The listing builds one solid part. Answer for the finished solid, in the listing's coordinates (mm). Face numbers are marked on the shaded views. A direction names the side the tool comes from. Give positions to 0.01 mm unless a question says otherwise; leave off trailing zeros. Write each loop counter-clockwise with the first axis right and the second up, starting at its lowest first coordinate (ties: lowest second). Pieces come first, ordered by that corner, then holes. Notation, with made-up numbers: (-1, -26) - (55, -26) arc R27 cw to (55, 3) - close; hole circle Ø1 at (-25.5, 80.25). An arc over 180 degrees is marked (long way). Answer as CSV lines item,"result". Start each with the question number.
(1) Find section B-B (z = 0). Write down the section's boundary in (x, y) (3 decimals), then the cut area to 3 significant figures.
(2) Straight lines are drawn through the part: probe 1 along Z at (x, y) = (-0.5, -4); probe 2 along X at (y, z) = (-6.5, 0); probe 3 along X at (y, z) = (108.73, 17.25). For each, find the intervals that lie inside material, in ascending order.
(3) Each of these flat-tipped pins is pushed along its axis until it touches: pin 1 Ø2.5 at (x, z) = (-20, -28) entering from -Y; pin 2 Ø1 at (x, z) = (14, -2.5) entering from +Y; pin 3 Ø17 at (y, z) = (89.5, 13.5) entering from +X. Where does it stop, or does it pass through?
(4) For a pull along Y with two mould halves and no side action, classify the marked faces 6, 7 and 8 as pulls with the +Y half, pulls with the -Y half, needs draft (parallel to the pull), parting line crosses it, or undercut.
(5) For the marked faces 1, 2, 3, 4 and 5, determine the directions among +Z, -Z, +X, -X, +Y, -Y from which every point of the face is accessible in a straight line to the end or side of a thin tool.
(6) Find section D-D (y = 3). Write down the section's boundary in (x, z).
(7) Find section C-C (y = 28.5). Write down the section's boundary in (x, z).
(8) Find section A-A (z = -30.68). Write down the section's boundary in (x, y).
from build123d import *

# Parameters (mm, degrees)
SKETCH_1_R           = 20.68
SKETCH_1_R_2         = 9.68
EXTRUDE_1_DEPTH      = 116.68
SKETCH_11_W          = 27
SKETCH_11_H          = 150
CUT_EXTRUDE_3_DEPTH  = 40
SKETCH_13_W          = 10
SKETCH_13_H          = 128.345013401
CUT_EXTRUDE_7_DEPTH  = 126.614916312
SKETCH_15_W          = 8
SKETCH_15_H          = 68.68
CUT_EXTRUDE_9_DEPTH  = 48
SKETCH_16_W          = 15.549431524
SKETCH_16_H          = 20
SKETCH_16_W_2        = 15.459431524
EXTRUDE_4_DEPTH      = 19.2
SKETCH_17_W          = 19.20851187
SKETCH_17_H          = 14.03
CUT_EXTRUDE_10_DEPTH = 20.2
SKETCH_18_R          = 9.59
CUT_EXTRUDE_11_DEPTH = 121.289430957
SKETCH_21_R          = 2.985
CUT_EXTRUDE_12_DEPTH = 55.2
EXTRUDE_START        = 55.2
SKETCH_24_R          = 20.59
SKETCH_24_R_2        = 9.59
EXTRUDE_2_DEPTH      = 55.2
CUT_EXTRUDE_13_DEPTH = 55.2
SKETCH_26_W          = 10.00851187
SKETCH_26_H          = 41.68
CUT_EXTRUDE_15_DEPTH = 55.2
SKETCH_27_W          = 10
SKETCH_27_H          = 40
CUT_EXTRUDE_16_DEPTH = 55.2
SKETCH_28_W          = 44.880694938
SKETCH_28_H          = 9.608044066
CUT_EXTRUDE_17_DEPTH = 12.2
SKETCH_35_W          = 13.53
SKETCH_35_H          = 20
EXTRUDE_10_DEPTH     = 15
EXTRUDE_11_DEPTH     = 15
SKETCH_37_W          = 9
SKETCH_37_H          = 20
EXTRUDE_12_DEPTH     = 20
SKETCH_38_W          = 9
SKETCH_38_H          = 20
EXTRUDE_13_DEPTH     = 20
SKETCH_42_R          = 2.985
CUT_EXTRUDE_21_DEPTH = 20


with BuildPart() as part:
    # 草圖1 → 伸長-薄件1 (new body)
    with BuildSketch(Plane(origin=(0, 0, 0), x_dir=(1, 0, 0), z_dir=(0, 1, 0))):
        Circle(SKETCH_1_R)
        Circle(SKETCH_1_R_2, mode=Mode.SUBTRACT)
    extrude(amount=EXTRUDE_1_DEPTH)

    # 草圖11 → 除料-伸長3 (cut)
    with BuildSketch(Plane(origin=(0, 116.68, 0), x_dir=(1, 0, 0), z_dir=(0, 1, 0))):
        with Locations((21.70851187, -44.235815192)):
            Rectangle(SKETCH_11_W, SKETCH_11_H)
    extrude(amount=-CUT_EXTRUDE_3_DEPTH, mode=Mode.SUBTRACT)

    # 草圖13 → 除料-伸長7 (cut, through all)
    with BuildSketch(Plane.XY.offset(21)):
        with Locations((-16, 58.612182466)):
            Rectangle(SKETCH_13_W, SKETCH_13_H)
    extrude(amount=-CUT_EXTRUDE_7_DEPTH, mode=Mode.SUBTRACT)

    # 草圖15 → 除料-伸長9 (cut)
    with BuildSketch(Plane.XY.offset(21)):
        with Locations((-1.395744065, 52.34)):
            Rectangle(SKETCH_15_W, SKETCH_15_H)
    extrude(amount=-CUT_EXTRUDE_9_DEPTH, mode=Mode.SUBTRACT)

    # 草圖16 → 填料-伸長4 (add)
    with BuildSketch(Plane(origin=(8.20851187, 0, 0), x_dir=(0, 0, -1), z_dir=(1, 0, 0))):
        with Locations((12.905284238, 106.68)):
            Rectangle(SKETCH_16_W, SKETCH_16_H)
        with Locations((-12.860284238, 106.68)):
            Rectangle(SKETCH_16_W_2, SKETCH_16_H)
    extrude(amount=-EXTRUDE_4_DEPTH)

    # 草圖17 → 除料-伸長10 (cut)
    with BuildSketch(Plane(origin=(0, 116.68, 0), x_dir=(1, 0, 0), z_dir=(0, 1, 0))):
        with Locations((-1.395744065, -0.045)):
            Rectangle(SKETCH_17_W, SKETCH_17_H)
    extrude(amount=-CUT_EXTRUDE_10_DEPTH, mode=Mode.SUBTRACT)

    # 草圖18 → 除料-伸長11 (cut, through all)
    with BuildSketch(Plane.XZ):
        with Locations(Location((0, 0, 0), (0, 0, 90))):
            Circle(SKETCH_18_R)
    extrude(amount=-CUT_EXTRUDE_11_DEPTH, mode=Mode.SUBTRACT)

    # 草圖21 → 除料-伸長12 (cut)
    with BuildSketch(Plane(origin=(0, 0, -20.68), x_dir=(-1, 0, 0), z_dir=(0, 0, -1))):
        with Locations((1.39148813, 108.73)):
            Circle(SKETCH_21_R)
    extrude(amount=-CUT_EXTRUDE_12_DEPTH, mode=Mode.SUBTRACT)

    # 草圖24 → 伸長-薄件2 (add)
    with BuildSketch(Plane.XZ.offset(EXTRUDE_START)):
        Circle(SKETCH_24_R)
        Circle(SKETCH_24_R_2, mode=Mode.SUBTRACT)
    extrude(amount=-EXTRUDE_2_DEPTH)

    # 草圖25 → 除料-伸長13 (cut)
    with BuildSketch(Plane.XY.offset(21)):
        Polygon((-1.39148813, -11.785), (22.612379708, -11.785), (22.612379708, -63.873337429), (-22.749525245, -63.873337429), (-22.749525245, -11.785), align=None)
    extrude(amount=-CUT_EXTRUDE_13_DEPTH, mode=Mode.SUBTRACT)

    # 草圖26 → 除料-伸長15 (cut)
    with BuildSketch(Plane(origin=(0, 0, 0), x_dir=(1, 0, 0), z_dir=(0, 1, 0))):
        with Locations((-15.995744065, -0.16)):
            Rectangle(SKETCH_26_W, SKETCH_26_H)
    extrude(amount=-CUT_EXTRUDE_15_DEPTH, mode=Mode.SUBTRACT)

    # 草圖27 → 除料-伸長16 (cut)
    with BuildSketch(Plane(origin=(21, 0, 0), x_dir=(0, 0, -1), z_dir=(1, 0, 0))):
        with Locations((0, 41.68)):
            Rectangle(SKETCH_27_W, SKETCH_27_H)
    extrude(amount=-CUT_EXTRUDE_16_DEPTH, mode=Mode.SUBTRACT)

    # 草圖28 → 除料-伸長17 (cut)
    with BuildSketch(Plane(origin=(21, 0, 0), x_dir=(0, 0, -1), z_dir=(1, 0, 0))):
        Rectangle(SKETCH_28_W, SKETCH_28_H)
    extrude(amount=-CUT_EXTRUDE_17_DEPTH, mode=Mode.SUBTRACT)

    # 草圖35 → 填料-伸長10 (add)
    with BuildSketch(Plane.ZY.offset(10.99148813)):
        with Locations((13.825, 106.68)):
            Rectangle(SKETCH_35_W, SKETCH_35_H)
    extrude(amount=EXTRUDE_10_DEPTH)

    # 草圖36 → 填料-伸長11 (add)
    with BuildSketch(Plane.ZY.offset(10.99148813)):
        Polygon((-20.68, 116.68), (-6.97, 116.68), (-6.97, 96.48), (-20.68, 96.68), align=None)
    extrude(amount=EXTRUDE_11_DEPTH)

    # 草圖37 → 填料-伸長12 (add)
    with BuildSketch(Plane.XY.offset(20.59)):
        with Locations((-21.49148813, 106.68)):
            Rectangle(SKETCH_37_W, SKETCH_37_H)
    extrude(amount=EXTRUDE_12_DEPTH)

    # 草圖38 → 填料-伸長13 (add)
    with BuildSketch(Plane(origin=(0, 0, -20.68), x_dir=(-1, 0, 0), z_dir=(0, 0, -1))):
        with Locations((21.49148813, 106.68)):
            Rectangle(SKETCH_38_W, SKETCH_38_H)
    extrude(amount=EXTRUDE_13_DEPTH)

    # 草圖42 → 除料-伸長21 (cut)
    with BuildSketch(Plane(origin=(-16.99148813, 0, 0), x_dir=(0, 0, -1), z_dir=(1, 0, 0))):
        with Locations((30.68, 106.554418142)):
            Circle(SKETCH_42_R)
        with Locations((-30.395640125, 106.68)):
            Circle(SKETCH_42_R)
    extrude(amount=-CUT_EXTRUDE_21_DEPTH, mode=Mode.SUBTRACT)


solid = part.part
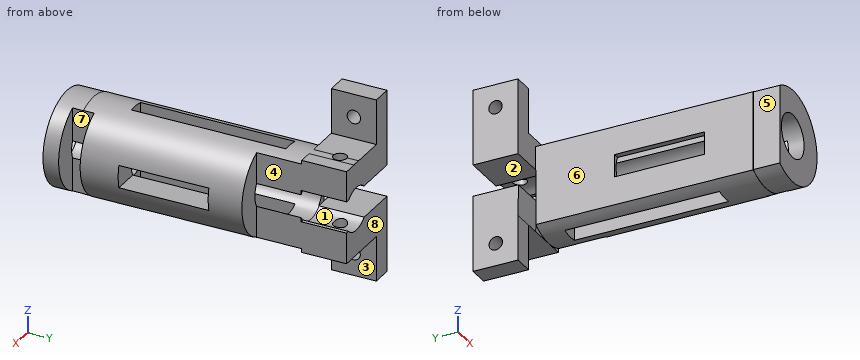
Result set:
1,outline,"(-11, 0) - (-10.991, 0) - (-10.991, -11.785) - (-9.59, -11.785) - (-9.59, 0) - (-9.68, 0) - (-9.68, 21.68) - (-11, 21.68) - close; (-11, 61.68) - (-9.68, 61.68) - (-9.68, 96.48) - (-11, 96.48) - close; (9.59, -11.785) - (20.59, -11.785) - (20.59, -4.804) - (9.59, -4.804) - close; (9.68, 4.804) - (20.68, 4.804) - (20.68, 21.68) - (9.68, 21.68) - close; (9.68, 61.68) - (20.68, 61.68) - (20.68, 76.68) - (9.68, 76.68) - close"
1,area,"518 mm^2"
2,probe 1,"-20.58 to -9.58, 9.58 to 20.58"
2,probe 2,"-10.99 to -9.59, 9.59 to 20.59"
2,probe 3,"-25.99 to -4.38, 1.59 to 8.21"
3,pin 1,"y = 96.68"
3,pin 2,"y = 76.68"
3,pin 3,"x = 8.21"
4,face 6,"needs draft"
4,face 7,"undercut"
4,face 8,"pulls with the +Y half"
5,face 1,"+Y, -Y"
5,face 2,"+X, -X, +Y"
5,face 3,"-Z, +X, +Y, -Y"
5,face 4,"+Z, -Z, +X, +Y"
5,face 5,"+Z, -Z, -X, -Y"
6,outline,"(-11, -17.51) arc R20.68 ccw to (8.8, -18.71) - (8.8, -4.03) arc R9.68 cw (long way) to (8.8, 4.03) - (8.8, 18.71) arc R20.68 ccw to (-11, 17.51) - close"
7,outline,"(-11, -17.51) arc R20.68 ccw to (-5.4, -19.96) - (-5.4, -8.04) arc R9.68 cw to (-8.29, -5) - (-11, -5) - close; (-11, 5) - (-8.29, 5) arc R9.68 cw to (-5.4, 8.04) - (-5.4, 19.96) arc R20.68 ccw to (-11, 17.51) - close; (2.6, -20.52) arc R20.68 ccw to (20.07, -5) - (8.29, -5) arc R9.68 cw to (2.6, -9.32) - close; (2.6, 9.32) arc R9.68 cw to (8.29, 5) - (20.07, 5) arc R20.68 ccw to (2.6, 20.52) - close"
8,outline,"(-25.99, 96.68) - (-16.99, 96.68) - (-16.99, 103.57) - (-25.99, 103.57) - close; (-25.99, 109.54) - (-16.99, 109.54) - (-16.99, 116.68) - (-25.99, 116.68) - close"
